Source: CAD feature listing. Evaluate the final solid. Frame: model axes, mm. Face numbers are marked on the shaded views. A direction names the side the tool comes from. Round coordinates to 2 decimals unless told otherwise and drop trailing zeros. Write each loop counter-clockwise with the first axis right and the second up, starting at its lowest first coordinate (ties: lowest second). Pieces come first, ordered by that corner, then holes.
```python
from build123d import *

# Parameters (mm, degrees)
F0_W     = 100
F0_H     = 50
F1_DEPTH = 50
F2_R     = 6.5
F3_DEPTH = 50.001
F4_DEPTH = 13
F7_DEPTH = 13
F9_DEPTH = 25


with BuildPart() as f1:
    # F0 (on Right) → F1 (new body)
    with BuildSketch(Plane.YZ):
        with Locations((50, 25)):
            Rectangle(F0_W, F0_H)
    extrude(amount=-F1_DEPTH)

    # F2 (on face) → F3 (cut, through all)
    with BuildSketch(Plane.YZ):
        with Locations((87, 25)):
            Circle(F2_R)
    extrude(amount=-F3_DEPTH, mode=Mode.SUBTRACT)

    # F2 (on face) → F4 (cut)
    with BuildSketch(Plane.YZ):
        Polygon((32, 25), (75, 50), (0, 50), (0, 25), align=None)
    extrude(amount=-F4_DEPTH, mode=Mode.SUBTRACT)

    # F6 (on face) → F7 (cut)
    with BuildSketch(Plane(origin=(-50, 0, 0), x_dir=(0, -1, 0), z_dir=(-1, 0, 0))):
        Polygon((-32, 25), (0, 25), (0, 50), (-75, 50), align=None)
    extrude(amount=-F7_DEPTH, mode=Mode.SUBTRACT)

    # F8 (on face) → F9 (cut)
    with BuildSketch(Plane(origin=(-37, 0, 0), x_dir=(0, -1, 0), z_dir=(-1, 0, 0))):
        Polygon((-54.36, 38), (0, 38), (0, 50), (-75, 50), align=None)
    extrude(amount=-F9_DEPTH, mode=Mode.SUBTRACT)


solid = f1.part
```
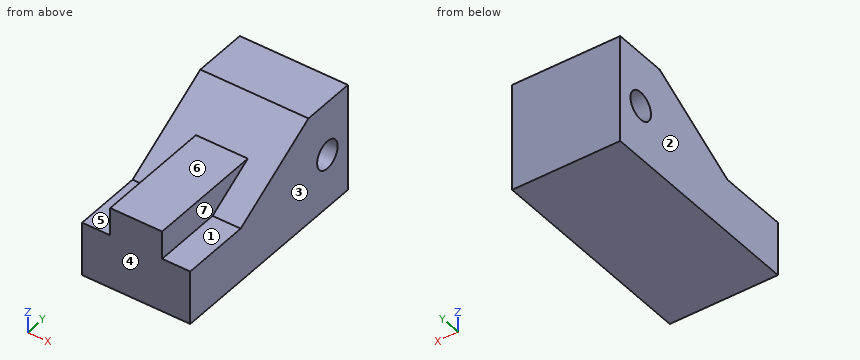
Q1. Line query: line 1 (Z direction, x = -17, y = 87); line 2 (Z direction, x = -47.5, y = 27.5); line 3 (X direction, y = 19.5, z = 35). Output: solid intervals per line, ascending.
Q2. Pin query (flat end, axial travel): P1, Ø4, axis at y = 37.5, z = 34, coming from the +X side; P2, Ø6, axis at x = -20.5, y = 29.5, coming from the +Z side; P3, Ø10.5, axis at x = -44.5, y = 10, coming from the +Z side. Return the tip coordinate at first contact, or that it passes through.
Q3. Section query C-C, the plane z = 26. Output: boundary loops of the cut face in (x, y).
Q4. Set-up query: the marked faces 4, 5, 6 and 7. Return all of +Z, -Z, +X, -X, +Y, -Y with unobstructed straight access to the full face (end or side cutting, diameter ignored); none if empty.
Q5. Mould query, pull axis X, two halves, no side actions, for the marked faces 1, 2 and 3. Classes: pulls with the +X half, pulls with the -X half, needs draft (parallel to the pull), parting line crosses it, or undercut.
Q6. Section query A-A, the plane y = 87. Output: boundary loops of the cut face in (x, z).
Q7. Section query B-B, the plane x = -42. Output: boundary loops of the cut face in (y, z), and give its area (3 significant figures).
Q8. Section query D-D, the plane x = -22. Output: boundary loops of the cut face in (y, z).
Filled in:
1. line 1: z = 0 to 18.5, 31.5 to 50
1. line 2: z = 0 to 25
1. line 3: x = -37 to -13
2. P1: stops at x = -13
2. P2: stops at z = 38
2. P3: stops at z = 25
3. outline: (-50, 33.72) - (-37, 33.72) - (-37, 0) - (-13, 0) - (-13, 33.72) - (0, 33.72) - (0, 80.58) - (-50, 80.58) - close; (-50, 93.42) - (0, 93.42) - (0, 100) - (-50, 100) - close
4. face 4: +Z, -Z, +X, -X, -Y
4. face 5: +Z, -X, -Y
4. face 6: +Z, +X, -X, -Y
4. face 7: +Z, +X, -Y
5. face 1: needs draft
5. face 2: pulls with the -X half
5. face 3: pulls with the +X half
6. outline: (-50, 0) - (0, 0) - (0, 18.5) - (-50, 18.5) - close; (-50, 31.5) - (0, 31.5) - (0, 50) - (-50, 50) - close
7. outline: (0, 0) - (100, 0) - (100, 50) - (75, 50) - (32, 25) - (0, 25) - close; hole circle Ø13 at (87, 25)
7. area: 3,530 mm2
8. outline: (0, 0) - (100, 0) - (100, 50) - (75, 50) - (54.36, 38) - (0, 38) - close; hole circle Ø13 at (87, 25)
